Design review of the part shown in the three views and the two pictorial views. Dimensions are in mm from the part's minimum x, y and z. Coordinates: 2 decimals unless noted, no trailing zeros. Loops run counter-clockwise (first coordinate to the right, second up) from the corner with the lowest first, then second, coordinate; pieces in that order, holes last. Notation, with made-up numbers: M 44.25,-23 L 103.25,-23 A24 cw 103.25,13 Z; hole C -34.75,-6 d8. An arc over 180 degrees is marked long. Answer as a JSON object with one key per item and string values. Group by question number.
Item 1: Add section B-B (z = 0.2). State the section outline as (x, y) points, then the cut area to 3 significant figures.
Item 2: Mouldability with a two-part tool opening along X and no side actions: class the marked faces 1, 2 and 3 as +X half, -X half, draft (parallel to the pull), parting line (faces both ways), or undercut.
Item 3: Wall thickness on L1, parallel to X at y = 4.75, z = 0.9; L2, parallel to Y at x = 0.85, z = 0.85; L3, parallel to X at y = 5.25, z = 0.75: over which ranges is each line inside the solid? List them lowest first. Write a range as from..to.
Item 4: Add section D-D (x = 1.3). State the section outline as (y, z) points.
Item 5: Add section A-A (x = 2.4). State the section outline as (y, z) points, then the cut area to 3 significant figures.
Item 6: Add section C-C (y = 0.75). State the section outline as (x, z) points.
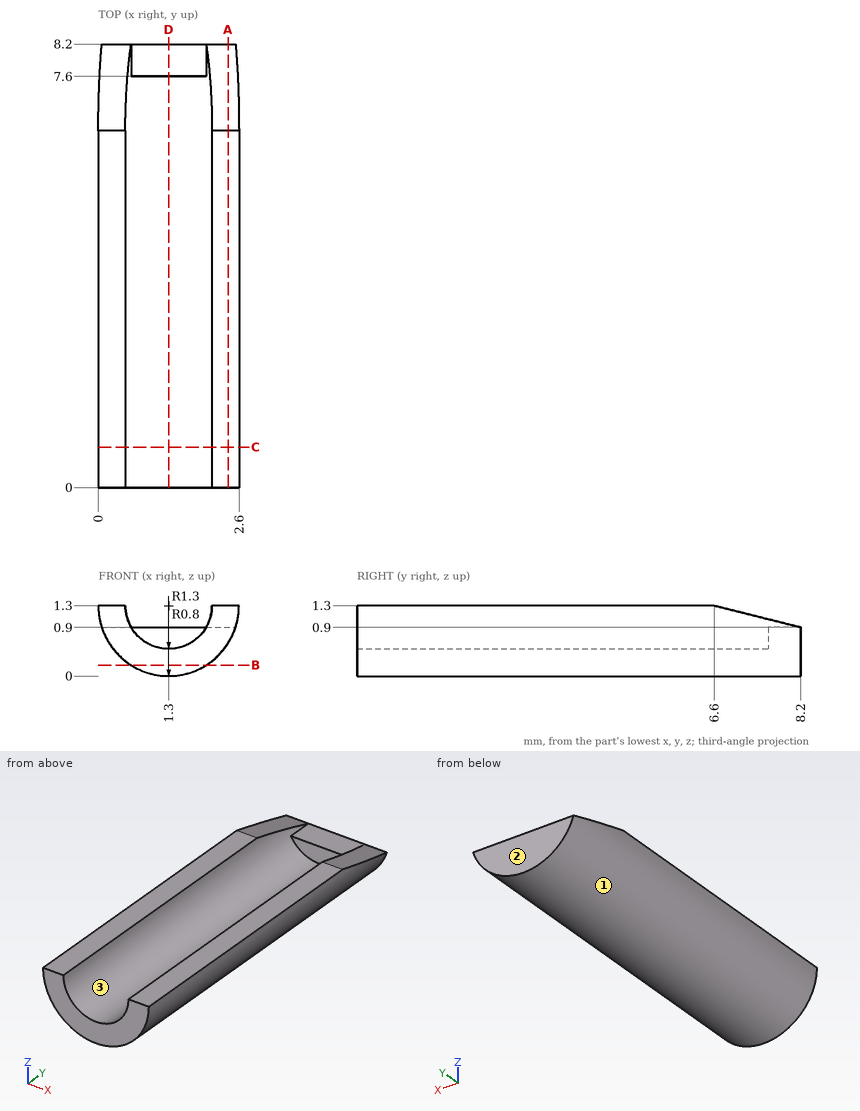
From the geometry:
{
 "1": {"outline": "M 0.61,0 L 1.99,0 L 1.99,8.2 L 0.61,8.2 Z", "area": "11.4 mm²"},
 "2": {"face 1": "parting line", "face 2": "draft", "face 3": "undercut"},
 "3": {"L1": "x = 0.06..0.61, 1.99..2.54", "L2": "y = 7.6..8.2", "L3": "x = 0.12..0.72, 1.88..2.48"},
 "4": {"outline": "M 0,0 L 8.2,0 L 8.2,0.9 L 7.6,0.9 L 7.6,0.5 L 0,0.5 Z"},
 "5": {"outline": "M 0,0.61 L 8.2,0.61 L 8.2,0.9 L 6.6,1.3 L 0,1.3 Z", "area": "5.36 mm²"},
 "6": {"outline": "M 0,1.3 A1.3 ccw 2.6,1.3 L 2.1,1.3 A0.8 cw 0.5,1.3 Z"}
}
